Geometry check sheet. Reference: the model listing, model coordinates, mm. A direction names the side the tool comes from. Give positions to 0.01 mm unless a question says otherwise; leave off trailing zeros. Loops run counter-clockwise (first coordinate to the right, second up) from the corner with the lowest first, then second, coordinate; pieces in that order, holes last. Notation, with made-up numbers: (30, 17) - (37, 17) arc R4 ccw to (37, 24) - close; hole circle Ø11 at (10.25, 18). An arc over 180 degrees is marked (long way). Use a Markdown table: item, result. Add a question column.
1. Draft check along Z on faces 1 (the cylindrical face through (12.52, -15.87, -0.35)), 2 (the flat face through (13, 26, -15.875)), 3 (the flat face through (13, -104, -508)), 4 (the flat face through (13, 50.8, 258)). Enter one of: pulls with the +Z half, pulls with the -Z half, needs draft (parallel to the pull), parting line crosses it, or undercut.
2. Depth check by flat-ended pin: P1, Ø10, axis at y = -194.5, z = 357.5, coming from the -X side. Enter the tip coordinate at first touch or a pass-through.
3. Set-up check for faces 5 (the flat face through (0, -99, 7)), 6 (the flat face through (13, 25, 15.875)): record each of +Z, -Z, +X, -X, +Y, -Y from which the full face is reachable in a straight line by a thin tool's end or side.
4. Cross-section at A-A on z = 0. Enter the section's corners in (x, y) (3 decimals), and give its area (3 significant figures).
5. Material ranges on L1, parallel to Y at x = 1.75, z = 0.5, recorded low to high.
from build123d import *

# Parameters (mm, degrees)
BOSS_EXTRUDE1_DEPTH = 25.4


with BuildPart() as part:
    # Sketch1 → Boss-Extrude1 (new body)
    with BuildSketch(Plane(origin=(0, 0, 0), x_dir=(0, 0, -1), z_dir=(1, 0, 0))):
        with BuildLine():
            ThreePointArc((15.875, 0), (0, -15.875), (-15.875, 0))
            Line((-15.875, 0), (-15.875, 50.8))
            Line((-15.875, 50.8), (-508, 50.8))
            Line((-508, 50.8), (-508, -254))
            Line((-508, -254), (508, -254))
            Line((508, -254), (508, 50.8))
            Line((508, 50.8), (15.875, 50.8))
            Line((15.875, 50.8), (15.875, 0))
        make_face()
    extrude(amount=BOSS_EXTRUDE1_DEPTH)


solid = part.part
Values found:
| question | item | result |
|---|---|---|
| 1 | face 1 | undercut |
| 1 | face 2 | undercut |
| 1 | face 3 | pulls with the -Z half |
| 1 | face 4 | needs draft |
| 2 | P1 | stops at x = 0 |
| 3 | face 5 | +Z, -Z, -X, +Y, -Y |
| 3 | face 6 | +X, -X, +Y |
| 4 | outline | (0, -254) - (25.4, -254) - (25.4, -15.875) - (0, -15.875) - close |
| 4 | area | 6,050 mm2 |
| 5 | L1 | y = -254 to -15.87 |
